Can you work these out from the model? Positions are in its coordinate system, mm. A direction names the side the tool comes from. Coordinates: 2 decimals unless noted, no trailing zeros. Loops run counter-clockwise (first coordinate to the right, second up) from the corner with the lowest first, then second, coordinate; pieces in that order, holes last. Notation, with made-up numbers: M 89.5,-32.5 L 101.5,-32.5 A25 cw 101.5,-10.5 Z; hole C 72.25,9 d9. An arc over 180 degrees is marked long. Answer as a JSON object with one key per item and string values. Group by question number.
Item 1: Suppose I cut it at B-B (z = 0.25). Count the separate pieces of the cut face and the enclosed holes in it, then the cut area to 3 significant figures.
Item 2: Suppose I cut it at A-A (x = -8.89). Write out the boundary of the cut face in (y, z).
Item 3: Which directions (+Z, -Z, +X, -X, +Y, -Y) give clear straight access to the entire face, cutting with the end or side of a thin tool? Please do faces 5 (the flat face through (0, -5.08, 4)), 6 (the flat face through (0, 0, 0.7)), 7 (the flat face through (12, 0, 7.95)).
Item 4: We'd pull the mould along X, two halves only. Please class faces 1 (the flat face through (6, 0, 7.95)), 2 (the flat face through (-12.7, 0, 4)), 3 (the flat face through (4, 0, 7.95)), 4 (the flat face through (0, 0, 8)): +X half, -X half, draft (parallel to the pull), parting line (faces both ways), or undercut.
Item 5: If I drill on line 1 (Z direction, x = 5.25, y = 1.75); line 2 (Y direction, x = 4, z = -3.25); line 3 (Y direction, x = -10.5, z = 0.5), over which ranges is the centre line in solid material (lowest first)?
```python
from build123d import *

# Parameters (mm, degrees)
SKETCH_W        = 25.4
SKETCH_H        = 10.16
PAD_DEPTH       = 8
SKETCH001_W     = 1.8
SKETCH001_H     = 5.1
POCKET_DEPTH    = 0.05
CHAMFER_SIZE    = 0.7
POCKET001_DEPTH = 10.161
POCKET002_DEPTH = 25.401
SKETCH004_R     = 0.25
PAD001_DEPTH    = 4.7


with BuildPart() as part:
    # Sketch → Pad (new body)
    with BuildSketch(Plane.XY):
        Rectangle(SKETCH_W, SKETCH_H)
    extrude(amount=PAD_DEPTH)

    # Sketch001 (on Face6 of Pad) → Pocket (cut)
    with BuildSketch(Plane.XY.offset(8)):
        with Locations((-11.52, 0)):
            Rectangle(SKETCH001_W, SKETCH001_H)
        with Locations((-6.4, 0)):
            Rectangle(SKETCH001_W, SKETCH001_H)
        with Locations((-3.84, 0)):
            Rectangle(SKETCH001_W, SKETCH001_H)
        with Locations((-1.28, 0)):
            Rectangle(SKETCH001_W, SKETCH001_H)
        with Locations((1.28, 0)):
            Rectangle(SKETCH001_W, SKETCH001_H)
        with Locations((3.84, 0)):
            Rectangle(SKETCH001_W, SKETCH001_H)
        with Locations((6.4, 0)):
            Rectangle(SKETCH001_W, SKETCH001_H)
        with Locations((8.96, 0)):
            Rectangle(SKETCH001_W, SKETCH001_H)
        with Locations((11.52, 0)):
            Rectangle(SKETCH001_W, SKETCH001_H)
        with Locations((-8.96, 0)):
            Rectangle(SKETCH001_W, SKETCH001_H)
    extrude(amount=-POCKET_DEPTH, mode=Mode.SUBTRACT)

    # Chamfer
    chamfer_edges = [part.edges().sort_by_distance(p)[0] for p in [
        (-12.7, -5.08, 4),
    ]]
    chamfer(chamfer_edges, length=CHAMFER_SIZE)

    # Sketch002 (on Face6 of Chamfer) → Pocket001 (cut, through all)
    with BuildSketch(Plane.XZ.offset(5.08)):
        Polygon((-10.16, 0), (-9.755855, 0.7), (9.755855, 0.7), (10.16, 0), align=None)
    extrude(amount=-POCKET001_DEPTH, mode=Mode.SUBTRACT)

    # Sketch003 (on Face11 of Pocket001) → Pocket002 (cut, through all)
    with BuildSketch(Plane.YZ.offset(12.7)):
        Polygon((-2.42, 0), (-2.015855, 0.7), (2.015855, 0.7), (2.42, 0), align=None)
    extrude(amount=-POCKET002_DEPTH, mode=Mode.SUBTRACT)

    # Sketch004 (on Face58 of Pocket002) → Pad001 (join)
    with BuildSketch(Plane(origin=(0, 0, 0.7), x_dir=(1, 0, 0), z_dir=(0, 0, -1))):
        with Locations((-11.43, 3.75)):
            Circle(SKETCH004_R)
        with Locations((-8.89, 3.75)):
            Circle(SKETCH004_R)
        with Locations((-6.35, 3.75)):
            Circle(SKETCH004_R)
        with Locations((-3.81, 3.75)):
            Circle(SKETCH004_R)
        with Locations((-1.27, 3.75)):
            Circle(SKETCH004_R)
        with Locations((1.27, 3.75)):
            Circle(SKETCH004_R)
        with Locations((3.81, 3.75)):
            Circle(SKETCH004_R)
        with Locations((6.35, 3.75)):
            Circle(SKETCH004_R)
        with Locations((8.89, 3.75)):
            Circle(SKETCH004_R)
        with Locations((11.43, 3.75)):
            Circle(SKETCH004_R)
        with Locations((-11.43, -3.75)):
            Circle(SKETCH004_R)
        with Locations((-8.89, -3.75)):
            Circle(SKETCH004_R)
        with Locations((-6.35, -3.75)):
            Circle(SKETCH004_R)
        with Locations((-3.81, -3.75)):
            Circle(SKETCH004_R)
        with Locations((-1.27, -3.75)):
            Circle(SKETCH004_R)
        with Locations((1.27, -3.75)):
            Circle(SKETCH004_R)
        with Locations((3.81, -3.75)):
            Circle(SKETCH004_R)
        with Locations((6.35, -3.75)):
            Circle(SKETCH004_R)
        with Locations((8.89, -3.75)):
            Circle(SKETCH004_R)
        with Locations((11.43, -3.75)):
            Circle(SKETCH004_R)
    extrude(amount=PAD001_DEPTH)


solid = part.part
```
From the geometry:
{
 "1": {"separate pieces": "20", "enclosed holes": "0", "area": "33.0 mm2"},
 "2": {"outline": "M -5.08,0.7 L -4,0.7 L -4,-4 L -3.5,-4 L -3.5,0.7 L 3.5,0.7 L 3.5,-4 L 4,-4 L 4,0.7 L 5.08,0.7 L 5.08,8 L 2.55,8 L 2.55,7.95 L -2.55,7.95 L -2.55,8 L -5.08,8 Z"},
 "3": {"face 5": "+Z, -Z, +X, -X, -Y", "face 6": "-Z", "face 7": "+Z"},
 "4": {"face 1": "undercut", "face 2": "-X half", "face 3": "undercut", "face 4": "draft"},
 "5": {"line 1": "0.7 to 8", "line 2": "-3.91 to -3.59, 3.59 to 3.91", "line 3": "-5.08 to -2.13, 2.13 to 5.08"}
}
